```python
from build123d import *

# Parameters (mm, degrees)
F1_DEPTH        = 4
F2_W            = 32
F2_H            = 36
F3_DEPTH        = 18
F5_DEPTH        = 32
F2_W_2          = 20
F2_H_2          = 25
F6_DEPTH        = 20
F7_R            = 4.25
F8_DEPTH        = 25
F9_W            = 2.8
F9_H            = 5.8
F10_DEPTH       = 12
F11_R           = 1.6
F12_DEPTH       = 10
F13_T1_DEPTH    = 4
F13_T3_DEPTH    = 34
F13_T5_DEPTH    = 54
F2_W_3          = 8.8
F2_H_3          = 2.4
F14_DEPTH       = 20
F15_R           = 1.6
F16_DEPTH       = 22
F18_D           = 3.3
F18_CSINK_D     = 6.72
F18_CSINK_ANGLE = 90
F19_R           = 1.2


# Not quite as in the source:
# - a fillet or chamfer that OpenCascade refuses, or shapes differently, is made with other operations: its cross-section is extruded or revolved along the edge and cut away or added


with BuildPart() as f1:
    # F0 (on Top) → F1 (new body)
    with BuildSketch(Plane.XY):
        Polygon((-45, -40), (-15, -40), (-15, -10), (45, -10), (45, 40), (-45, 40), align=None)
    extrude(amount=F1_DEPTH)

    # F2 (on face) → F3 (join)
    with BuildSketch(Plane.XY.offset(4)):
        with Locations((0, 18)):
            Rectangle(F2_W, F2_H)
    extrude(amount=F3_DEPTH)

    # F4 (on face) → F5 (cut, through all)
    with BuildSketch(Plane.YZ.offset(16)):
        with BuildLine():
            ThreePointArc((4.4707723798, 22), (16.1846745035, 4.5181920003), (32, 18.4))
            ThreePointArc((32, 18.4), (31.8818079997, 20.2153254965), (31.5292276202, 22))
            Line((31.5292276202, 22), (4.4707723798, 22))
        make_face()
    extrude(amount=-F5_DEPTH, mode=Mode.SUBTRACT)

    # F2 (on face) → F6 (join)
    with BuildSketch(Plane.XY.offset(4)):
        with Locations((-35, -27.5)):
            Rectangle(F2_W_2, F2_H_2)
    extrude(amount=F6_DEPTH)

    # F7 (on face) → F8 (cut, through all)
    with BuildSketch(Plane.XZ.offset(40)):
        with Locations((-35, 18.4)):
            Circle(F7_R)
    extrude(amount=-F8_DEPTH, mode=Mode.SUBTRACT)

    # F9 (on face) → F10 (cut)
    with BuildSketch(Plane.XY.offset(24)):
        with Locations((-42.4, -27.5)):
            Rectangle(F9_W, F9_H)
    extrude(amount=-F10_DEPTH, mode=Mode.SUBTRACT)

    # F11 (on face) → F12 (cut)
    with BuildSketch(Plane(origin=(-45, 0, 0), x_dir=(0, -1, 0), z_dir=(-1, 0, 0))):
        with Locations((27.5, 18.4)):
            Circle(F11_R)
    extrude(amount=-F12_DEPTH, mode=Mode.SUBTRACT)

    # F13: fillet of radius 6 on 6 edges, made by hand

    # F13_s2 → F13_t1 (join)
    with BuildSketch(Plane.XY):
        with BuildLine():
            ThreePointArc((-15, -16), (-13.2426406871, -11.7573593129), (-9, -10))
            Line((-9, -10), (-15, -10))
            Line((-15, -10), (-15, -16))
        make_face()
    extrude(amount=F13_T1_DEPTH)

    # F13_s4 → F13_t3 (cut)
    with BuildSketch(Plane.XY.offset(-15)):
        with BuildLine():
            ThreePointArc((-21, -40), (-16.7573593129, -38.2426406871), (-15, -34))
            Line((-15, -34), (-15, -40))
            Line((-15, -40), (-21, -40))
        make_face()
        with BuildLine():
            ThreePointArc((39, -10), (43.2426406871, -8.2426406871), (45, -4))
            Line((45, -4), (45, -10))
            Line((45, -10), (39, -10))
        make_face()
        with BuildLine():
            ThreePointArc((39, 40), (43.2426406871, 38.2426406871), (45, 34))
            Line((45, 34), (45, 40))
            Line((45, 40), (39, 40))
        make_face()
        with BuildLine():
            ThreePointArc((-45, 34), (-43.2426406871, 38.2426406871), (-39, 40))
            Line((-39, 40), (-45, 40))
            Line((-45, 40), (-45, 34))
        make_face()
    extrude(amount=F13_T3_DEPTH, mode=Mode.SUBTRACT)

    # F13_s6 → F13_t5 (cut)
    with BuildSketch(Plane.XY.offset(-15)):
        with BuildLine():
            ThreePointArc((-39, -40), (-43.2426406871, -38.2426406871), (-45, -34))
            Line((-45, -34), (-45, -40))
            Line((-45, -40), (-39, -40))
        make_face()
    extrude(amount=F13_T5_DEPTH, mode=Mode.SUBTRACT)

    # F2 (on face) → F14 (join)
    with BuildSketch(Plane.XY.offset(4)):
        Polygon((36.2, 23.6), (36.2, 26), (33.8, 26), (33.8, 4), (36.2, 4), (36.2, 6.4), align=None)
        with Locations((40.6, 5.2)):
            Rectangle(F2_W_3, F2_H_3)
        with Locations((40.6, 24.8)):
            Rectangle(F2_W_3, F2_H_3)
    extrude(amount=F14_DEPTH)

    # F15 (on face) → F16 (cut, through all)
    with BuildSketch(Plane.XZ.offset(-4)):
        with Locations((39.4, 14)):
            Circle(F15_R)
    extrude(amount=-F16_DEPTH, mode=Mode.SUBTRACT)

    # F18 (through all)
    with Locations(Plane(origin=(0, 0, 0), x_dir=(1, 0, 0), z_dir=(0, 0, -1))):
        with Locations((-21, 34), (39, 4), (39, -34), (-39, -34)):
            CounterSinkHole(F18_D / 2, F18_CSINK_D / 2, counter_sink_angle=F18_CSINK_ANGLE)

    # F19
    f19_edges = [f1.edges().sort_by_distance(p)[0] for p in [
        (0, 40, 0),
        (-43.242641, 38.242641, 0),
        (-30, -40, 0),
        (-43.242641, -38.242641, 0),
        (-45, 0, 0),
        (43.242641, 38.242641, 0),
        (45, 15, 0),
        (-16.757359, -38.242641, 0),
        (43.242641, -8.242641, 0),
        (-15, -25, 0),
        (15, -10, 0),
        (-13.242641, -11.757359, 0),
    ]]
    fillet(f19_edges, radius=F19_R)


solid = f1.part
```
Work out the finished part from the listing and answer in its coordinate system (mm). A direction names the side the tool comes from. Give positions to 0.01 mm unless a question says otherwise; leave off trailing zeros. Order: outer loops, then holes, each group sorted by start corner. A loop starts at its lowest first (then second) coordinate and runs counter-clockwise, first axis right, second up.
1. Each of these flat-tipped pins is pushed along its axis until it touches: P1, Ø2, axis at x = -8.5, z = 10.5, coming from the +Y side; P2, Ø8, axis at x = 16, y = -14.5, coming from the +Z side; P3, Ø6, axis at y = -26.5, z = 15.5, coming from the +X side; P4, Ø4, axis at x = 39.4, z = 14, coming from the -Y side. Where does it stop, or does it pass through?
Result sheet:
P1: stops at y = 36
P2: passes through
P3: stops at x = -25
P4: stops at y = 4
2. The mould has two halves that part along X. Classify faces 1 (the flat face through (16, 13.7, 4.9)), 2 (the flat face through (-25, -28, 14)), 3 (the flat face through (-1, 9, 0)), 4 (the cylindrical face through (40.216, 32.885, 2.871)): released by +X, released by -X, zero draft, split by the parting line, or undercut.
Result sheet:
face 1: undercut
face 2: released by +X
face 3: zero draft
face 4: undercut
3. Section A-A, the plane y = -27.5 is taken. Determine the outline of the cut face in (x, z), and give its area (3 significant figures).
Result sheet:
outline: (-45, 1.2) arc R1.2 ccw to (-43.8, 0) - (-16.2, 0) arc R1.2 ccw to (-15, 1.2) - (-15, 4) - (-25, 4) - (-25, 24) - (-41, 24) - (-41, 20) - (-38.94, 20) arc R4.25 cw (long way) to (-38.94, 16.8) - (-41, 16.8) - (-41, 12) - (-43.8, 12) - (-43.8, 16.8) - (-45, 16.8) - close; (-45, 20) - (-43.8, 20) - (-43.8, 24) - (-45, 24) - close
area: 419 mm2
4. Section B-B, the plane z = 9.5 is taken. Determine the outline of the cut face in (x, y), and give its area (3 significant figures).
Result sheet:
outline: (-45, -34) arc R6 ccw to (-39, -40) - (-25, -40) - (-25, -15) - (-45, -15) - close; (-16, 0) - (16, 0) - (16, 7.19) - (-16, 7.19) - close; (-16, 28.81) - (16, 28.81) - (16, 36) - (-16, 36) - close; (33.8, 4) - (45, 4) - (45, 6.4) - (36.2, 6.4) - (36.2, 23.6) - (45, 23.6) - (45, 26) - (33.8, 26) - close
area: 1,050 mm2
5. Straight lines are drawn through the part: L1, parallel to Y at x = 39, z = 3.05; L2, parallel to Y at x = 40, z = 8; L3, parallel to Y at x = 9, z = 19. For each, find the intervals that lie inside material, in ascending order.
Result sheet:
L1: y = -10 to -5.65, -2.35 to 32.35, 35.65 to 40
L2: y = 4 to 6.4, 23.6 to 26
L3: y = 0 to 4.01, 31.99 to 36
6. Section D-D, the plane z = 21 is taken. Give the number of separate pieces and of enclosed holes in the cut face, and give its area (3 significant figures).
Result sheet:
separate pieces: 5
enclosed holes: 1
area: 675 mm2
7. For faces 5 (the flat face through (-16, 13.7, 4.9)), 6 (the flat face through (-35.1, -15, 13.9)), 7 (the cylindrical face through (-44.41, -26.23, 17.43)), determine the directions among +Z, -Z, +X, -X, +Y, -Y from which every point of the face is accessible in a straight line to the end or side of a thin tool.
Result sheet:
face 5: +Z, -X, +Y, -Y
face 6: +Z, +X, -X, +Y
face 7: -X
8. Section C-C, the plane y = -17 is taken. Determine the outline of the cut face in (x, z), and give its area (3 significant figures).
Result sheet:
outline: (-45, 1.2) arc R1.2 ccw to (-43.8, 0) - (-16.2, 0) arc R1.2 ccw to (-15, 1.2) - (-15, 4) - (-25, 4) - (-25, 24) - (-45, 24) - close; hole circle Ø8.5 at (-35, 18.4)
area: 463 mm2
